from build123d import *

# Parameters (mm, degrees)
F2_DEPTH = 82
F1_W     = 1.6
F1_H     = 10
F3_DEPTH = 10
F4_START = -72
F4_DEPTH = 10
F6_W     = 1.6
F6_H     = 10
F7_DEPTH = 10
F8_START = 102.8
F8_DEPTH = 10


with BuildPart() as f2:
    # F1 (on offset) → F2 (new body)
    with BuildSketch(Plane.XZ.offset(41)):
        Polygon((78.5, 0), (78.5, 1.6), (-78.5, 1.6), (-78.5, 0), (-76.9, 0), (-74.1, 0), (-72.5, 0), (-40.3, 0), (-38.7, 0), (-35.9, 0), (-34.3, 0), (34.3, 0), (35.9, 0), (38.7, 0), (40.3, 0), (72.5, 0), (74.1, 0), (76.9, 0), align=None)
    extrude(amount=-F2_DEPTH)

    # F1 (on offset) → F3 (join)
    with BuildSketch(Plane.XZ.offset(41)):
        with Locations((-77.7, -5)):
            Rectangle(F1_W, F1_H)
        with Locations((-73.3, -5)):
            Rectangle(F1_W, F1_H)
        with Locations((-39.5, -5)):
            Rectangle(F1_W, F1_H)
        with Locations((-35.1, -5)):
            Rectangle(F1_W, F1_H)
        with Locations((35.1, -5)):
            Rectangle(F1_W, F1_H)
        with Locations((39.5, -5)):
            Rectangle(F1_W, F1_H)
        with Locations((73.3, -5)):
            Rectangle(F1_W, F1_H)
        with Locations((77.7, -5)):
            Rectangle(F1_W, F1_H)
    extrude(amount=-F3_DEPTH)

    # F1 (on offset) → F4 (join)
    with BuildSketch(Plane.XZ.offset(41).offset(F4_START)):
        with Locations((-77.7, -5)):
            Rectangle(F1_W, F1_H)
        with Locations((-73.3, -5)):
            Rectangle(F1_W, F1_H)
        with Locations((-39.5, -5)):
            Rectangle(F1_W, F1_H)
        with Locations((-35.1, -5)):
            Rectangle(F1_W, F1_H)
        with Locations((39.5, -5)):
            Rectangle(F1_W, F1_H)
        with Locations((35.1, -5)):
            Rectangle(F1_W, F1_H)
        with Locations((73.3, -5)):
            Rectangle(F1_W, F1_H)
        with Locations((77.7, -5)):
            Rectangle(F1_W, F1_H)
    extrude(amount=-F4_DEPTH)

    # F6 (on offset) → F7 (join)
    with BuildSketch(Plane.YZ.offset(-51.4)):
        with Locations((-10.3, -5)):
            Rectangle(F6_W, F6_H)
        with Locations((-17.1, -5)):
            Rectangle(F6_W, F6_H)
    extrude(amount=-F7_DEPTH)

    # F6 (on offset) → F8 (join)
    with BuildSketch(Plane.YZ.offset(-51.4).offset(F8_START)):
        with Locations((-10.3, -5)):
            Rectangle(F6_W, F6_H)
        with Locations((-17.1, -5)):
            Rectangle(F6_W, F6_H)
    extrude(amount=F8_DEPTH)


solid = f2.part
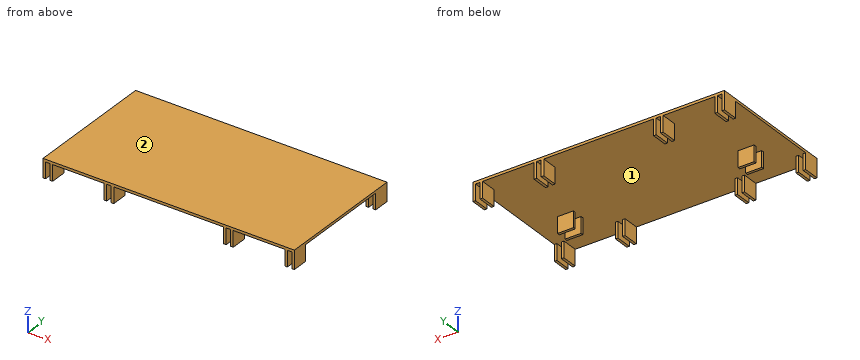
Can you work these out from the model? Positions are in its coordinate system, mm. Face numbers are marked on the shaded views. Coordinates: 2 decimals unless noted, no trailing zeros. Write each loop counter-clockwise with the first axis right and the second up, starting at its lowest first coordinate (ties: lowest second). Pieces come first, ordered by that corner, then holes. Notation, with made-up numbers: (27, 5) - (50, 5) arc R35 cw to (50, 38) - close; hole circle Ø11 at (70.5, 58). An arc over 180 degrees is marked (long way). Return JSON: item names as keys, results as strings. Group by question number.
Item 1: We'd pull the mould along X, two halves only. Please class the marked faces 1 and 2: pulls with the +X half, pulls with the -X half, needs draft (parallel to the pull), parting line crosses it, or undercut.
Item 2: If we section it at D-D (x = 13.5): Write out the boundary of the cut face in (y, z).
Item 3: If we section it at C-C (z = -1.75): Count the separate pieces of the cut face and the enclosed holes in it, then the cut area to 3 significant figures.
Item 4: If we section it at A-A (x = -54.5): Write out the boundary of the cut face in (y, z), then the cut area to 3 significant figures.
Item 5: Please list where these lines run through material, in increasing order: probe 1 along Y at (x, z) = (-61, -9.5); probe 2 along Z at (x, y) = (-36, -8).
Item 6: I'm going to push flat-ended pins straight in: pin 1 Ø10 at (x, y) = (15.5, 28.5) entering from -Z; pin 2 Ø0.8 at (y, z) = (-17, -2.5) entering from -X; pin 3 Ø3 at (x, z) = (-58.5, -4.5) entering from +Y. Where does each tip first touch, or does it pass through?
Return value:
{
 "1": {"face 1": "undercut", "face 2": "needs draft"},
 "2": {"outline": "(-41, 0) - (41, 0) - (41, 1.6) - (-41, 1.6) - close"},
 "3": {"separate pieces": "20", "enclosed holes": "0", "area": "320 mm^2"},
 "4": {"outline": "(-41, 0) - (-17.9, 0) - (-17.9, -10) - (-16.3, -10) - (-16.3, 0) - (-11.1, 0) - (-11.1, -10) - (-9.5, -10) - (-9.5, 0) - (41, 0) - (41, 1.6) - (-41, 1.6) - close", "area": "163 mm^2"},
 "5": {"probe 1": "y = -17.9 to -16.3, -11.1 to -9.5", "probe 2": "z = 0 to 1.6"},
 "6": {"pin 1": "stops at z = 0", "pin 2": "stops at x = -61.4", "pin 3": "stops at y = -9.5"}
}
